Autodesk Inventor part; units mm, degrees
ref_plane "YZ Plane" through (0, 0, 0) normal (1, 0, 0) x (0, 1, 0)
ref_plane "XZ Plane" through (0, 0, 0) normal (0, 1, 0) x (-1, 0, 0)
ref_plane "XY Plane" through (0, 0, 0) normal (0, 0, 1) x (1, 0, 0)
sketch "Esboço1" plane through (0, 0, 0) normal (0, 1, 0) x (-1, 0, 0)
  line L0 (-30.5, -18.5) -> (30.5, -18.5)
  line L1 (30.5, -18.5) -> (30.5, 18.5)
  line L2 (30.5, 18.5) -> (-30.5, 18.5)
  line L3 (-30.5, 18.5) -> (-30.5, -18.5)
  line L4 (-30.5, -18.5) -> (30.5, 18.5) construction
  line L5 (30.5, -18.5) -> (-30.5, 18.5) construction
  point P0 (0, 0)
  point P1 (0, 0)
  dimension "d2" = 61
  dimension "d3" = 37
  dimension "d6" = 0
  dimension "d7" = 0
extrude "Extrusão1" add sketch "Esboço1" along normal blind 5
sketch "Esboço3" plane through (0, 5, 0) normal (0, 1, 0) x (1, 0, 0)
  line L0 (29, -17) -> (-29, -17)
  line L1 (-29, -17) -> (-29, 17)
  line L2 (-29, 17) -> (29, 17)
  line L3 (29, 17) -> (29, -17)
  line L4 (29, -17) -> (-29, 17) construction
  line L5 (-29, -17) -> (29, 17) construction
  line L6 (-30.5, 18.5) -> (-30.5, -18.5)
  line L7 (30.5, -18.5) -> (-30.5, -18.5)
  line L8 (-30.5, -18.5) -> (-30.5, 18.5)
  line L9 (-30.5, 18.5) -> (30.5, 18.5)
  line L10 (30.5, 18.5) -> (30.5, -18.5)
  line L11 (30.5, -18.5) -> (-30.5, 18.5) construction
  line L12 (-30.5, -18.5) -> (30.5, 18.5) construction
  point P0 (0, 0)
  point P1 (-30.5, -18.5)
  dimension "d49" = 1.5
  dimension "d50" = 1.5
extrude "Extrusão2" add sketch "Esboço3" along normal blind 8
chamfer "Chanfro1" distance 2 angle 45 4 edges at (-30.5, 6.5, -18.5) (-30.5, 6.5, 18.5) (30.5, 6.5, 18.5) (30.5, 6.5, -18.5)
chamfer "Chanfro2" distance 2 angle 45 4 edges at (29, 9, 17) (-29, 9, 17) (29, 9, -17) (-29, 9, -17)
sketch "Esboço4" plane through (0, 0, 0) normal (0, -1, 0) x (1, 0, 0)
  line L0 (26.5, 15.5) -> (-26.5, 15.5)
  line L1 (-26.5, 15.5) -> (-26.5, 10.5)
  line L2 (-26.5, 10.5) -> (26.5, 10.5)
  line L3 (26.5, 10.5) -> (26.5, 15.5)
  line L4 (-30.5, 18.5) -> (30.5, 18.5)
  line L5 (-30.5, -18.5) -> (-30.5, 18.5)
  line L6 (30.5, 18.5) -> (30.5, -18.5)
  line L7 (-26.5, -15.5) -> (26.5, -15.5)
  line L8 (26.5, -15.5) -> (26.5, -10.5)
  line L9 (26.5, -10.5) -> (-26.5, -10.5)
  line L10 (-26.5, -10.5) -> (-26.5, -15.5)
  line L11 (30.5, -18.5) -> (-30.5, -18.5)
  point P0 (0, 0)
  point P1 (-28.5, 18.5)
  point P2 (28.5, 18.5)
  point P3 (-30.5, -16.5)
  point P4 (-30.5, 16.5)
  point P5 (30.5, 16.5)
  point P6 (30.5, -16.5)
  point P7 (26.5, 13)
  point P8 (26.5, -13)
  point P9 (-26.5, -13)
  point P10 (28.5, -18.5)
  point P11 (-28.5, -18.5)
  dimension "d18" = 3
  dimension "d19" = 5
  dimension "d20" = 4
  dimension "d21" = 4
  dimension "d23" = 4
  dimension "d24" = 4
  dimension "d25" = 5
  dimension "d26" = 3
extrude "Extrusão3" cut sketch "Esboço4" against normal through all contours L3 L2 L1 L0 | L10 L9 L8 L7
sketch "Esboço5" plane through (0, 0, 0) normal (0, -1, 0) x (1, 0, 0)
  line L0 (26.5, 10.5) -> (-26.5, 10.5)
  line L1 (-26.5, 10.5) -> (-26.5, 15.5)
  line L2 (-26.5, 15.5) -> (26.5, 15.5)
  line L3 (26.5, 15.5) -> (26.5, 10.5)
  line L4 (-26.5, -10.5) -> (26.5, -10.5)
  line L5 (26.5, -10.5) -> (26.5, -15.5)
  line L6 (26.5, -15.5) -> (-26.5, -15.5)
  line L7 (-26.5, -15.5) -> (-26.5, -10.5)
  line L8 (30.5, 16.5) -> (30.5, -16.5)
  line L9 (-28.5, 18.5) -> (28.5, 18.5)
  line L10 (-30.5, -16.5) -> (-30.5, 16.5)
  line L11 (28.5, -18.5) -> (-28.5, -18.5)
  circle A0 centre (15, 8) radius 1.5
  circle A1 centre (15, -8) radius 1.5
  circle A2 centre (-15, 8) radius 1.5
  circle A3 centre (-15, -8) radius 1.5
  line L12 (17.5, 10.5) -> (-17.5, 10.5)
  line L13 (-17.5, 10.5) -> (-17.5, -10.5)
  line L14 (-17.5, -10.5) -> (17.5, -10.5)
  line L15 (17.5, -10.5) -> (17.5, 10.5)
  line L16 (17.5, 10.5) -> (-17.5, -10.5) construction
  line L17 (-17.5, 10.5) -> (17.5, -10.5) construction
  line L18 (30.5, -16.5) -> (28.5, -18.5)
  line L19 (28.5, 18.5) -> (30.5, 16.5)
  line L20 (-30.5, 16.5) -> (-28.5, 18.5)
  line L21 (-28.5, -18.5) -> (-30.5, -16.5)
  circle A4 centre (-7.65, 5.5) radius 1.5
  circle A5 centre (7.65, 5.5) radius 1.5
  point P0 (0, 0)
  dimension "d31" = 3
  dimension "d35" = 2.5
  dimension "d36" = 2.5
  dimension "d38" = 2.5
  dimension "d42" = 35
  dimension "d43" = 2.5
  dimension "d44" = 2.5
  dimension "d45" = 21
  dimension "d46" = 2.5
  dimension "d47" = 2.5
  dimension "d48" = 2.5
  dimension "d51" = 3
  dimension "d52" = 3
  dimension "d55" = 5
  dimension "d56" = 5
  dimension "d58" = 15.3
  dimension "d59" = 9.85
  dimension "d60" = 9.85
extrude "Extrusão4" cut sketch "Esboço5" against normal through all contours A0 | A1 | A2 | A3 | A4 | A5
equation "\"d59\" = d60"
properties part number "espTopLayer"
Geometry check sheet. Reference: the model listing, model coordinates, mm. A direction names the side the tool comes from. Give positions to 0.01 mm unless a question says otherwise; leave off trailing zeros. Loops run counter-clockwise (first coordinate to the right, second up) from the corner with the lowest first, then second, coordinate; pieces in that order, holes last. Notation, with made-up numbers: M -26,52 L -9,52 A29 ccw -9,87 Z; hole C 10,-10.5 d1. An arc over 180 degrees is marked long. Answer as CSV lines item,"result".
Item 1: Cross-section at B-B on y = 9.75. Record the cut outline in (x, z), and give its area (3 significant figures).
Values:
outline,"M -30.5,-16.5 L -28.5,-18.5 L 28.5,-18.5 L 30.5,-16.5 L 30.5,16.5 L 28.5,18.5 L -28.5,18.5 L -30.5,16.5 Z; hole M -29,-15 L -27,-17 L 27,-17 L 29,-15 L 29,15 L 27,17 L -27,17 L -29,15 Z"
area,"285 mm²"
Item 2: Cross-section at A-A on x = -7.65. Record the cut outline in (y, z), and give its area (3 significant figures).
Values:
outline,"M 0,-18.5 L 13,-18.5 L 13,-17 L 5,-17 L 5,-15.5 L 0,-15.5 Z; M 0,-10.5 L 5,-10.5 L 5,4 L 0,4 Z; M 0,7 L 5,7 L 5,10.5 L 0,10.5 Z; M 0,15.5 L 5,15.5 L 5,17 L 13,17 L 13,18.5 L 0,18.5 Z"
area,"144 mm²"
Item 3: Depth check by flat-ended pin: P1, Ø3.5, axis at x = -15, z = 8, coming from the +Y side; P2, Ø2.5, axis at x = 7.65, z = 5.5, coming from the +Y side. Enter the tip coordinate at first touch or a pass-through.
Values:
P1,"stops at y = 5"
P2,"passes through"
Item 4: Access from +Z, -Z, +X, -X, +Y, -Y to the whole of each face (thin tool, end or side, straight path). Record for faces 5 (the flat face through (0, 0, 0)), 6 (the flat face through (0, 2, 10.5)), 7 (the flat face through (-28, 9, 16)).
Values:
face 5,"+Z, -Z, +X, -X, -Y"
face 6,"+Y, -Y"
face 7,"+Y"
Item 5: Release check for a two-part mould opening along X. For faces 1 (the cylindrical face through (-6.264, 2.465, 4.925)), 2 (the flat face through (0, 13, 18)), 3 (the flat face through (26.5, 2, -13)), 4 (the flat face through (-30, 7, -17)) record: pulls with the +X half, pulls with the -X half, needs draft (parallel to the pull), parting line crosses it, or undercut.
Values:
face 1,"undercut"
face 2,"needs draft"
face 3,"undercut"
face 4,"pulls with the -X half"
Item 6: Material ranges on line 1 (Z direction, x = 18.5, y = 2.25); line 2 (Z direction, x = -7.65, y = 2.55); line 3 (X direction, y = 7.25, z = -3), recorded low to high.
Values:
line 1,"z = -18.5 to -15.5, -10.5 to 10.5, 15.5 to 18.5"
line 2,"z = -18.5 to -15.5, -10.5 to 4, 7 to 10.5, 15.5 to 18.5"
line 3,"x = -30.5 to -29, 29 to 30.5"
Item 7: Cross-section at D-D on x = 15. Record the cut outline in (y, z).
Values:
outline,"M 0,-18.5 L 13,-18.5 L 13,-17 L 5,-17 L 5,-15.5 L 0,-15.5 Z; M 0,-10.5 L 5,-10.5 L 5,-9.5 L 0,-9.5 Z; M 0,-6.5 L 5,-6.5 L 5,6.5 L 0,6.5 Z; M 0,9.5 L 5,9.5 L 5,10.5 L 0,10.5 Z; M 0,15.5 L 5,15.5 L 5,17 L 13,17 L 13,18.5 L 0,18.5 Z"
Item 8: Cross-section at C-C on z = -8. Record the cut outline in (x, y).
Values:
outline,"M -30.5,0 L -16.5,0 L -16.5,5 L -29,5 L -29,13 L -30.5,13 Z; M -13.5,0 L 13.5,0 L 13.5,5 L -13.5,5 Z; M 16.5,0 L 30.5,0 L 30.5,13 L 29,13 L 29,5 L 16.5,5 Z"
